CAD build for the part. Positions are in the model's coordinates, mm. Round coordinates to 2 decimals unless told otherwise and drop trailing zeros. Order: outer loops, then holes, each group sorted by start corner. A loop starts at its lowest first (then second) coordinate and runs counter-clockwise, first axis right, second up. Notation, with made-up numbers: (58.25, 54.25) -> (82.25, 54.25) arc R15 ccw to (82.25, 59.25) -> close; hole circle Ø9 at (60, 9.5). An arc over 180 degrees is marked (long way). Return JSON: item names as keys, results as strings. Group by question number.
Q1. Flat gauge pin, fed straight in: pin 1 (6 mm diameter, centred on x = 66.29, y = -66.29, fed in from -Z). Where does the tip first touch, or does it go through?
Q2. Mould opens along X. For faces 1 (the cylindrical face through (-64.95, 64.18, 1.48)), 2 (the flat face through (-1, -79, 3)), 3 (the cylindrical face through (63.794, 66.181, 1.479)) say: +X half, -X half, draft (parallel to the pull), parting line (faces both ways), or undercut.
Q3. Probe line 1 along Y through (x, z) = (-64.5, 1.1); line 2 along Y through (x, z) = (10.5, 1.3); line 3 along Y through (x, z) = (28.5, 1.15). List the from-to ranges inside material, lowest first.
Q4. Cut at C-C (z = 1.05). Write the cut outline in (x, y), then the cut area to 3 significant figures.
Q5. Cut at A-A (y = 0). Write the cut outline in (x, z).
Q6. Cut at B-B (x = -50). Write the cut outline in (y, z), then the cut area to 3 significant figures.
Autodesk Inventor part; units mm, degrees
ref_plane "YZ Plane" through (0, 0, 0) normal (1, 0, 0) x (0, 1, 0)
ref_plane "XZ Plane" through (0, 0, 0) normal (0, 1, 0) x (-1, 0, 0)
ref_plane "XY Plane" through (0, 0, 0) normal (0, 0, 1) x (1, 0, 0)
sketch "スケッチ1" plane through (0, 0, 0) normal (0, 0, 1) x (1, 0, 0)
  line L0 (-100, 100) -> (100, 100)
  line L1 (100, 100) -> (100, -100)
  line L2 (100, -100) -> (-100, -100)
  line L3 (-100, -100) -> (-100, 100)
  line L4 (-100, 100) -> (100, -100) construction
  line L5 (100, 100) -> (-100, -100) construction
  circle A0 centre (0, 0) radius 93.75 construction
  circle A1 centre (-66.2913, 66.2913) radius 2.5
  circle A2 centre (66.2913, 66.2913) radius 2.5
  circle A3 centre (66.2913, -66.2913) radius 2.5
  circle A4 centre (-66.2913, -66.2913) radius 2.5
  dimension "d0" = 200
  dimension "d1" = 200
  dimension "d2" = 187.5
  dimension "d3" = 5
  dimension "d4" = 5
  dimension "d5" = 5
  dimension "d6" = 5
extrude "押し出し1" add sketch "スケッチ1" along normal blind 3
sketch "スケッチ2" plane through (0, 0, 0) normal (0, 0, -1) x (-1, 0, 0)
  circle A0 centre (0, 0) radius 72.5
  dimension "d9" = 145
extrude "押し出し2" cut sketch "スケッチ2" against normal blind 10
sketch "スケッチ3" plane through (0, 0, 3) normal (0, 0, 1) x (1, 0, 0)
  circle A0 centre (-66.2913, -66.2913) radius 2.5
  circle A1 centre (66.2913, -66.2913) radius 2.5
  point P0 (0, 0)
sketch "スケッチ4" plane through (-100, -100, 0) normal (0, -1, 0) x (1, 0, 0)
  line L0 (0, 0) -> (0, 3)
  line L1 (200, 0) -> (200, 3)
  line L2 (0, 3) -> (200, 3)
  line L3 (200, 3) -> (200, 0)
  line L4 (200, 0) -> (0, 0)
  line L5 (0, 0) -> (0, 3)
  point P0 (100, 0)
extrude "押し出し3" add sketch "スケッチ4" along normal blind 50
properties part number "ベアリング板" material "アルミニウム 6061"
Solution:
{
 "1": {"pin 1": "stops at z = 0"},
 "2": {"face 1": "undercut", "face 2": "draft", "face 3": "undercut"},
 "3": {"line 1": "y = -150 to -68.04, -64.55 to -33.11, 33.11 to 64.55, 68.04 to 100", "line 2": "y = -150 to -71.74, 71.74 to 100", "line 3": "y = -150 to -66.66, 66.66 to 100"},
 "4": {"outline": "(-100, -150) -> (100, -150) -> (100, 100) -> (-100, 100) -> close; hole circle Ø145 at (0, 0); hole circle Ø5 at (-66.29, -66.29); hole circle Ø5 at (-66.29, 66.29); hole circle Ø5 at (66.29, -66.29); hole circle Ø5 at (66.29, 66.29)", "area": "33,400 mm²"},
 "5": {"outline": "(-100, 0) -> (-72.5, 0) -> (-72.5, 3) -> (-100, 3) -> close; (72.5, 0) -> (100, 0) -> (100, 3) -> (72.5, 3) -> close"},
 "6": {"outline": "(-150, 0) -> (-52.5, 0) -> (-52.5, 3) -> (-150, 3) -> close; (52.5, 0) -> (100, 0) -> (100, 3) -> (52.5, 3) -> close", "area": "435 mm²"}
}
